Verification items for the finished model (mm, model axes). A direction names the side the tool comes from. Round coordinates to 2 decimals unless told otherwise and drop trailing zeros. Write each loop counter-clockwise with the first axis right and the second up, starting at its lowest first coordinate (ties: lowest second). Pieces come first, ordered by that corner, then holes.
from build123d import *

# Parameters (mm, degrees)
SKETCH_W         = 500
SKETCH_H         = 430
SKETCH_W_2       = 454
SKETCH_H_2       = 384
EXTRUDE_DEPTH    = 23
SKETCH001_W      = 23
SKETCH001_H      = 23
EXTRUDE001_DEPTH = 1554


with BuildPart() as extrude_body:
    # Sketch → Extrude (new body)
    with BuildSketch(Plane.YZ):
        with Locations((250, 215)):
            Rectangle(SKETCH_W, SKETCH_H)
        with Locations((250, 215)):
            Rectangle(SKETCH_W_2, SKETCH_H_2, mode=Mode.SUBTRACT)
    extrude(amount=EXTRUDE_DEPTH)


with BuildPart() as extrude001:
    # Clone base: copy of Extrude body
    add(extrude_body.part)


with BuildPart() as extrude001_1:
    # Clone placement: moved
    add(extrude001.part.moved(Location((1577, 0, 0))))


with BuildPart() as extrude002:
    # Sketch001 → Extrude001 (new body)
    with BuildSketch(Plane.YZ):
        with Locations((11.5, 11.5)):
            Rectangle(SKETCH001_W, SKETCH001_H)
    extrude(amount=EXTRUDE001_DEPTH)


with BuildPart() as extrude002_1:
    # Extrude001 placement: moved
    add(extrude002.part.moved(Location((23, 238.5, 0))))


with BuildPart() as extrude003:
    # Clone001 base: copy of Extrude002
    add(extrude002_1.part)


with BuildPart() as extrude003_1:
    # Clone001 placement: moved
    add(extrude003.part.moved(Location((0, -238.5, 407))))


with BuildPart() as extrude004:
    # Clone002 base: copy of Extrude003
    add(extrude003_1.part)


with BuildPart() as extrude004_1:
    # Clone002 placement: moved
    add(extrude004.part.moved(Location((0, 477, 0))))


with BuildPart() as fusion:
    # Fusion base: copy of Extrude body
    add(extrude_body.part)

    # Fusion: union Extrude001, Extrude002, Extrude003, Extrude004
    add(extrude001_1.part)
    add(extrude002_1.part)
    add(extrude003_1.part)
    add(extrude004_1.part)


solid = fusion.part
Q1. Depth check by flat-ended pin: P1, Ø18.5, axis at x = 841, z = 12.5, coming from the -Y side; P2, Ø7, axis at x = 1583, y = 191, coming from the -Z side. Enter the tip coordinate at first touch or a pass-through.
Recorded:
P1: stops at y = 238.5
P2: stops at z = 0
Q2. Material ranges on line 1 along Y through (x, z) = (114.5, 412.5), recorded low to high.
Recorded:
line 1: y = 0 to 23, 477 to 500
Q3. Sectioned sample at A-A (x = 1298.5). Enter the section's corners in (y, z).
Recorded:
outline: (0, 407) - (23, 407) - (23, 430) - (0, 430) - close; (238.5, 0) - (261.5, 0) - (261.5, 23) - (238.5, 23) - close; (477, 407) - (500, 407) - (500, 430) - (477, 430) - close
Q4. Sectioned sample at B-B (z = 146). Enter the section's corners in (x, y), plus the area to 3 significant figures.
Recorded:
outline: (0, 0) - (23, 0) - (23, 23) - (0, 23) - close; (0, 477) - (23, 477) - (23, 500) - (0, 500) - close; (1577, 0) - (1600, 0) - (1600, 23) - (1577, 23) - close; (1577, 477) - (1600, 477) - (1600, 500) - (1577, 500) - close
area: 2,120 mm2
Q5. Sectioned sample at C-C (y = 281.5). Enter the section's corners in (x, z).
Recorded:
outline: (0, 0) - (23, 0) - (23, 23) - (0, 23) - close; (0, 407) - (23, 407) - (23, 430) - (0, 430) - close; (1577, 0) - (1600, 0) - (1600, 23) - (1577, 23) - close; (1577, 407) - (1600, 407) - (1600, 430) - (1577, 430) - close
Q6. Tool access check on faces 1 (the flat face through (1577, 477.4, 144.2)), 2 (the flat face through (796, 490, 430)), 3 (the flat face through (1577, 22, 159)). Record the directions out of +Z, -Z, +X, -X, +Y, -Y that give a thin tool (end or side, any length) a straight path to the whole face; none if there is none.
Recorded:
face 1: -Z, +Y
face 2: +Z, +X, -X, +Y, -Y
face 3: -Z, -Y
